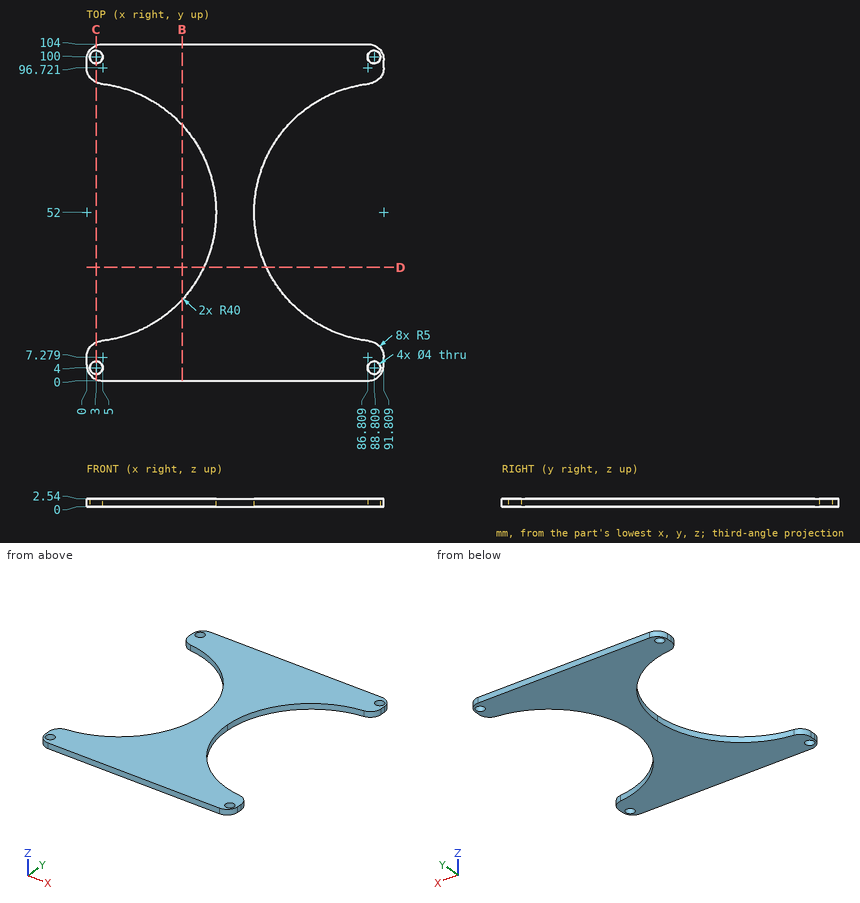
Verification items for this drawing (mm, ordinates from the low corner). Give positions to 0.01 mm unless a question says otherwise; leave off trailing zeros. Write each loop counter-clockwise with the first axis right and the second up, starting at its lowest first coordinate (ties: lowest second). Pieces come first, ordered by that corner, then holes. Notation, with made-up numbers: (20, 40.25) -> (69, 40.25) arc R24 ccw to (69, 72.25) -> close; hole circle Ø4 at (35, 67.5). An arc over 180 degrees is marked (long way). Use CSV: the item, a comma, the result in double quotes. Start each with the question number.
Q1. Depth check by flat-ended pin: P1, Ø2.5, axis at x = 3, y = 100, coming from the -Z side; P2, Ø1.5, axis at y = 21.5, z = 2, coming from the -X side; P3, Ø5, axis at x = 3, y = 4, coming from the +Z side. Enter the tip coordinate at first touch or a pass-through.
Q2. Cross-section at C-C on x = 3. Enter the section's corners in (y, z).
Q3. Cross-section at D-D on y = 35. Enter the section's corners in (x, z).
Q4. Scan lines: line 1 along X through (y, z) = (100, 1.25); line 2 along Y through (x, z) = (4.5, 0.2) (1 decimal); line 3 along Y through (x, z) = (3, 1.2). Record each from-to range of solid material in increasing order.
Q5. Cross-section at B-B on x = 29.5. Enter the section's corners in (y, z), and give its area (3 significant figures).
Working result:
1,P1,"passes through"
1,P2,"stops at x = 24.97"
1,P3,"stops at z = 2.54"
2,outline,"(0.42, 0) -> (2, 0) -> (2, 2.54) -> (0.42, 2.54) -> close; (6, 0) -> (11.86, 0) -> (11.86, 2.54) -> (6, 2.54) -> close; (92.14, 0) -> (98, 0) -> (98, 2.54) -> (92.14, 2.54) -> close; (102, 0) -> (103.58, 0) -> (103.58, 2.54) -> (102, 2.54) -> close"
3,outline,"(36.21, 0) -> (55.6, 0) -> (55.6, 2.54) -> (36.21, 2.54) -> close"
4,line 1,"x = 0.1 to 1, 5 to 86.81, 90.81 to 91.71"
4,line 2,"y = 0 to 2.7, 5.3 to 12.3, 91.7 to 98.7, 101.3 to 104"
4,line 3,"y = 0.42 to 2, 6 to 11.86, 92.14 to 98, 102 to 103.58"
5,outline,"(0, 0) -> (24.99, 0) -> (24.99, 2.54) -> (0, 2.54) -> close; (79.01, 0) -> (104, 0) -> (104, 2.54) -> (79.01, 2.54) -> close"
5,area,"127 mm^2"
